Here's how the part is built. I have some questions about the finished solid (model axes, mm). A direction names the side the tool comes from. Coordinates: 2 decimals unless noted, no trailing zeros. Write each loop counter-clockwise with the first axis right and the second up, starting at its lowest first coordinate (ties: lowest second). Pieces come first, ordered by that corner, then holes. Notation, with made-up numbers: (64, 85) -> (86, 85) arc R24 cw to (86, 104) -> close; hole circle Ø6 at (48, 52.25). An arc over 180 degrees is marked (long way). Use a Markdown table: item, result. Add a question column.
```python
from build123d import *

# Parameters (mm, degrees)
SKETCH1_W               = 14.5
SKETCH1_H               = 30
SKETCH1_R               = 3
BOSS_EXTRUDE1_DEPTH     = 5
CUT_EXTRUDE1_DEPTH      = 30.097274604
CUT_EXTRUDE1_DEPTH_BACK = 30.097274604
SKETCH2_R               = 4
CUT_EXTRUDE2_DEPTH      = 23.16293341
CUT_EXTRUDE2_DEPTH_BACK = 23.16293341
SKETCH3_R               = 3
CUT_EXTRUDE3_DEPTH      = 23.162933498
CUT_EXTRUDE3_DEPTH_BACK = 23.162933498
SKETCH4_R               = 3
BOSS_EXTRUDE5_START     = -10
SKETCH6_R               = 5
BOSS_EXTRUDE5_DEPTH     = 0.1
SKETCH7_R               = 0.4
BOSS_EXTRUDE6_DEPTH     = 9.9
SKETCH8_W               = 10
SKETCH8_H               = 5.416493121
CUT_EXTRUDE5_DEPTH      = 23.162933498
CUT_EXTRUDE6_START      = -10
CUT_EXTRUDE6_DEPTH      = 10
CUT_EXTRUDE7_START      = -14.5
CUT_EXTRUDE7_DEPTH      = 14.5


# Read off the part's stored shape, not the designer's step: Cut-Extrude6, Cut-Extrude7
with BuildPart() as part:
    # Sketch1 → Boss-Extrude1 (new, symmetric)
    with BuildSketch(Plane.XY):
        with Locations((-14.901879651, 0.998300452)):
            Rectangle(SKETCH1_W, SKETCH1_H)
        with Locations((-14.901879651, -4.732232083)):
            Circle(SKETCH1_R, mode=Mode.SUBTRACT)
    extrude(amount=BOSS_EXTRUDE1_DEPTH, both=True)

    # Sketch2 → Cut-Extrude1 (cut, two sides: drawn at the far end of the back side and taken through both)
    with BuildSketch(Plane(origin=(0, 0, -5), x_dir=(-1, 0, 0), z_dir=(0, 0, -1)).offset(-CUT_EXTRUDE1_DEPTH_BACK)):
        with Locations((14.901879651, -4.001699548)):
            Circle(SKETCH2_R)
    extrude(amount=CUT_EXTRUDE1_DEPTH + CUT_EXTRUDE1_DEPTH_BACK, mode=Mode.SUBTRACT)

    # Sketch3 → Cut-Extrude2 (cut, two sides: drawn at the far end of the back side and taken through both)
    with BuildSketch(Plane.ZY.offset(22.151879651).offset(-CUT_EXTRUDE2_DEPTH_BACK)):
        with Locations(Location((0, -8.608931628, 0), (0, 0, 270))):
            Circle(SKETCH3_R)
    extrude(amount=CUT_EXTRUDE2_DEPTH + CUT_EXTRUDE2_DEPTH_BACK, mode=Mode.SUBTRACT)

    # Sketch4 → Cut-Extrude3 (cut, two sides: drawn at the far end of the back side and taken through both)
    with BuildSketch(Plane.ZY.offset(22.151879651).offset(-CUT_EXTRUDE3_DEPTH_BACK)):
        with Locations(Location((0, 3.392776132, 0), (0, 0, 270))):
            Circle(SKETCH4_R)
    extrude(amount=CUT_EXTRUDE3_DEPTH + CUT_EXTRUDE3_DEPTH_BACK, mode=Mode.SUBTRACT)

    # Sketch6 → Boss-Extrude5 (add)
    with BuildSketch(Plane(origin=(0, 0, -5), x_dir=(-1, 0, 0), z_dir=(0, 0, -1)).offset(BOSS_EXTRUDE5_START)):
        with Locations((14.901879651, -4.001699548)):
            Circle(SKETCH6_R)
    extrude(amount=BOSS_EXTRUDE5_DEPTH)

    # Sketch7 → Boss-Extrude6 (add)
    with BuildSketch(Plane(origin=(0, 0, 4.9), x_dir=(-1, 0, 0), z_dir=(0, 0, -1))):
        with Locations(Location((14.901879651, -3.652232083, 0), (0, 0, 180))):
            Circle(SKETCH7_R)
    extrude(amount=BOSS_EXTRUDE6_DEPTH)

    # Sketch8 → Cut-Extrude5 (cut, through all)
    with BuildSketch(Plane(origin=(-7.651879651, 0, 0), x_dir=(0, 0, -1), z_dir=(1, 0, 0))):
        with Locations((0, 13.290053892)):
            Rectangle(SKETCH8_W, SKETCH8_H)
    extrude(amount=-CUT_EXTRUDE5_DEPTH, mode=Mode.SUBTRACT)

    # Cut-Extrude6 outline → Cut-Extrude6 (cut)
    with BuildSketch(Plane(origin=(0, 0, -5), x_dir=(-1, 0, 0), z_dir=(0, 0, -1)).offset(CUT_EXTRUDE6_START)):
        with BuildLine():
            ThreePointArc((7.651879651, 8.831200001), (9.341126693, 9.839033909), (11.162547128, 10.581807331))
            Line((11.162547128, 10.581807331), (7.651879651, 10.581807331))
            Line((7.651879651, 10.581807331), (7.651879651, 8.831200001))
        make_face()
        with BuildLine():
            Line((22.151879651, 10.581807331), (19.178996312, 10.581807331))
            ThreePointArc((19.178996312, 10.581807331), (20.709322329, 9.979718674), (22.151879651, 9.190138504))
            Line((22.151879651, 9.190138504), (22.151879651, 10.581807331))
        make_face()
        with BuildLine():
            ThreePointArc((10.371064905, -14.001699548), (8.967948653, -13.348856833), (7.651879651, -12.534669381))
            Line((7.651879651, -12.534669381), (7.651879651, -14.001699548))
            Line((7.651879651, -14.001699548), (10.371064905, -14.001699548))
        make_face()
        with BuildLine():
            Line((22.151879651, -14.001699548), (22.151879651, -12.893607884))
            ThreePointArc((22.151879651, -12.893607884), (21.087178214, -13.498835864), (19.970478535, -14.001699548))
            Line((19.970478535, -14.001699548), (22.151879651, -14.001699548))
        make_face()
    extrude(amount=CUT_EXTRUDE6_DEPTH, mode=Mode.SUBTRACT)

    # Cut-Extrude7 outline → Cut-Extrude7 (cut)
    with BuildSketch(Plane(origin=(-7.651879651, 0, 0), x_dir=(0, 0, -1), z_dir=(1, 0, 0)).offset(CUT_EXTRUDE7_START)):
        with BuildLine():
            ThreePointArc((5, -11.350842885), (0, -12.5864008), (-5, -11.350842885))
            Line((-5, -11.350842885), (-5, -14.001699548))
            Line((-5, -14.001699548), (5, -14.001699548))
            Line((5, -14.001699548), (5, -11.350842885))
        make_face()
        with BuildLine():
            Line((-5, 10.581807331), (-5, 7.647373505))
            ThreePointArc((-5, 7.647373505), (0, 8.882931421), (5, 7.647373505))
            Line((5, 7.647373505), (5, 10.581807331))
            Line((5, 10.581807331), (-5, 10.581807331))
        make_face()
    extrude(amount=CUT_EXTRUDE7_DEPTH, mode=Mode.SUBTRACT)


solid = part.part
```
Q1. Suppose I cut it at D-D, the plane y = -6. Write out the boundary of the cut face in (x, z), and give its area (3 significant figures).
Q2. Will these pins go through, and if not, where does the flat tip stop? pin 1 (3 mm diameter, centred on x = -17, z = 2.5, fed in from +Y); pin 2 (3 mm diameter, centred on x = -16, z = 2, fed in from -Y).
Q3. Which directions (+Z, -Z, +X, -X, +Y, -Y) give clear straight access to the entire face, cutting with the end or side of a thin tool? Please do faces 4 (the cylindrical face through (-15.2, -3.92, 0.02)), 5 (the flat face through (-22.152, -2, 0)).
Q4. Suppose I cut it at C-C, the plane z = 0. Write out the boundary of the cut face in (x, y).
Q5. Thinking about a two-plate mould opening in Y: for faces 1 (the cylindrical face through (-14.381, -0.036, 0.019)), 2 (the flat face through (-15, 0.4, 5)), 3 (the cylindrical face through (-15.003, 8.883, 0.073)), which applies, released by +Y, released by -Y, zero draft, split by the parting line, or undercut?
Q6. Suppose I cut it at B-B, the plane x = -10.5. Write out the boundary of the cut face in (y, z), and give its area (3 significant figures).
Q7. Please list where these lines run through material, in increasing order: line 1 (Y direction, x = -17.25, z = 0.5); line 2 (X direction, y = -3.75, z = 1.5); line 3 (Z direction, x = -12.75, y = 3.5).
Q8. Suppose I cut it at A-A, the plane y = 5.5. Write out the boundary of the cut face in (x, z), and give its area (3 significant figures).
Answer key:
| question | item | result |
|---|---|---|
| 1 | outline | (-22.15, -5) -> (-18.37, -5) -> (-18.37, -1.48) -> (-22.15, -1.48) -> close; (-22.15, 1.48) -> (-18.37, 1.48) -> (-18.37, 4.9) -> (-11.44, 4.9) -> (-11.44, 1.48) -> (-7.65, 1.48) -> (-7.65, 5) -> (-22.15, 5) -> close; (-11.44, -5) -> (-7.65, -5) -> (-7.65, -1.48) -> (-11.44, -1.48) -> close |
| 1 | area | 54.0 mm^2 |
| 2 | pin 1 | stops at y = 8.84 |
| 2 | pin 2 | stops at y = -12.57 |
| 3 | face 4 | -Z |
| 3 | face 5 | +Z, -Z, -X, +Y, -Y |
| 4 | outline | (-22.15, -12.59) -> (-7.73, -12.59) arc R13.06 ccw to (-7.65, -12.53) -> (-7.65, -11.61) -> (-22.15, -11.61) -> close; (-22.15, -5.61) -> (-18.56, -5.61) arc R4 cw (long way) to (-11.24, -5.61) -> (-7.65, -5.61) -> (-7.65, 0.39) -> (-22.15, 0.39) -> close; (-22.15, 6.39) -> (-7.65, 6.39) -> (-7.65, 8.83) arc R13.06 ccw to (-7.73, 8.88) -> (-22.15, 8.88) -> close; circle Ø0.8 at (-14.9, -3.65) |
| 5 | face 1 | undercut |
| 5 | face 2 | zero draft |
| 5 | face 3 | released by +Y |
| 6 | outline | (-11.35, -5) -> (7.65, -5) arc R10.73 ccw to (7.65, 5) -> (-11.35, 5) arc R10.73 ccw to start; hole circle Ø6 at (-8.61, 0); hole circle Ø6 at (3.39, 0) |
| 6 | area | 150 mm^2 |
| 7 | line 1 | y = -12.57 to -11.57, -0.76 to 0.43, 6.35 to 8.87 |
| 7 | line 2 | x = -22.15 to -18.89, -15.29 to -14.51, -10.91 to -7.65 |
| 7 | line 3 | z = -5 to -3, 3 to 5 |
| 8 | outline | (-22.15, -5) -> (-7.65, -5) -> (-7.65, -2.14) -> (-22.15, -2.14) -> close; (-22.15, 2.14) -> (-7.65, 2.14) -> (-7.65, 5) -> (-22.15, 5) -> close |
| 8 | area | 83.1 mm^2 |
